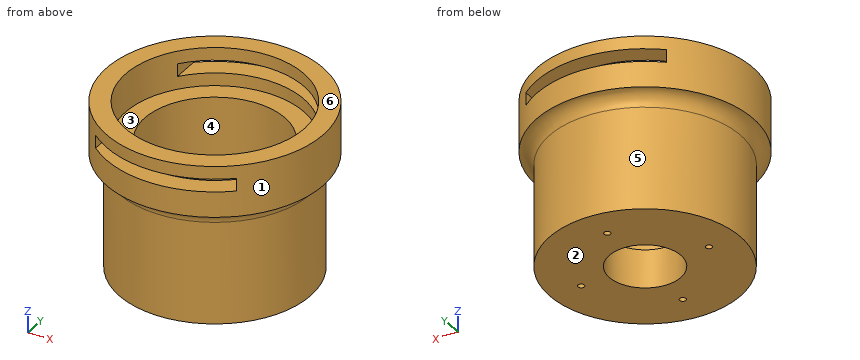
```python
from build123d import *

# Parameters (mm, degrees)
SKETCH1_R                = 15
BOSS_EXTRUDE5_DEPTH      = 26
SKETCH3_R                = 5.625
CUT_EXTRUDE2_DEPTH       = 34.555923471
CUT_EXTRUDE3_DEPTH       = 28
CUT_EXTRUDE3_DEPTH_BACK  = 20
SKETCH4_R                = 11
CUT_EXTRUDE6_START       = 6
SKETCH7_R                = 11
SKETCH7_R_2              = 9
CUT_EXTRUDE6_DEPTH       = 2
BOSS_EXTRUDE8_DEPTH      = 6
BOSS_EXTRUDE8_DEPTH_BACK = 2
BOSS_EXTRUDE8_START      = 20
SKETCH12_R               = 17
CUT_EXTRUDE10_START      = 18
SKETCH13_R               = 11
CUT_EXTRUDE10_DEPTH      = 18.411862419
FILLET2_R                = 2
CUT_EXTRUDE11_START      = 26
SKETCH14_R               = 14
CUT_EXTRUDE11_DEPTH      = 6
SKETCH15_R               = 0.5
CUT_EXTRUDE14_DEPTH      = 36.411862419
CUT_EXTRUDE15_DEPTH      = 36.411862419
CUT_EXTRUDE15_DEPTH_BACK = 36.411862419
SKETCH18_W               = 22
SKETCH18_H               = 2


with BuildPart() as part:
    # Sketch1 → Boss-Extrude5 (new body)
    with BuildSketch(Plane.XY):
        Circle(SKETCH1_R)
    extrude(amount=BOSS_EXTRUDE5_DEPTH)

    # Sketch3 → Cut-Extrude2 (cut, through all)
    with BuildSketch(Plane.XY.offset(26)):
        Circle(SKETCH3_R)
    extrude(amount=-CUT_EXTRUDE2_DEPTH, mode=Mode.SUBTRACT)

    # Sketch4 → Cut-Extrude3 (cut, two sides: drawn at the far end of the back side and taken through both)
    with BuildSketch(Plane.XY.offset(26).offset(-CUT_EXTRUDE3_DEPTH_BACK)):
        Circle(SKETCH4_R)
    extrude(amount=CUT_EXTRUDE3_DEPTH + CUT_EXTRUDE3_DEPTH_BACK, mode=Mode.SUBTRACT)

    # Sketch7 → Cut-Extrude6 (cut)
    with BuildSketch(Plane.XY.offset(CUT_EXTRUDE6_START)):
        Circle(SKETCH7_R)
        Circle(SKETCH7_R_2, mode=Mode.SUBTRACT)
    extrude(amount=-CUT_EXTRUDE6_DEPTH, mode=Mode.SUBTRACT)

    # Sketch12 → Boss-Extrude8 (add, two sides: drawn at the far end of the back side and taken through both)
    with BuildSketch(Plane.XY.offset(BOSS_EXTRUDE8_START - BOSS_EXTRUDE8_DEPTH_BACK)):
        Circle(SKETCH12_R)
    extrude(amount=BOSS_EXTRUDE8_DEPTH + BOSS_EXTRUDE8_DEPTH_BACK)

    # Sketch13 → Cut-Extrude10 (cut, through all)
    with BuildSketch(Plane.XY.offset(CUT_EXTRUDE10_START)):
        Circle(SKETCH13_R)
    extrude(amount=CUT_EXTRUDE10_DEPTH, mode=Mode.SUBTRACT)

    # Fillet2
    fillet2_edges = [part.edges().sort_by_distance(p)[0] for p in [
        (-15, 0, 18),
    ]]
    fillet(fillet2_edges, radius=FILLET2_R - 0.0001)  # a hair under: the kernel refuses the full size

    # Sketch14 → Cut-Extrude11 (cut)
    with BuildSketch(Plane.XY.offset(CUT_EXTRUDE11_START)):
        Circle(SKETCH14_R)
    extrude(amount=-CUT_EXTRUDE11_DEPTH, mode=Mode.SUBTRACT)

    # Sketch15 → Cut-Extrude14 (cut, through all)
    with BuildSketch(Plane.XY):
        with Locations((0, 10)):
            Circle(SKETCH15_R)
        with Locations((0, -10)):
            Circle(SKETCH15_R)
        with Locations((10, 0)):
            Circle(SKETCH15_R)
        with Locations((-10, 0)):
            Circle(SKETCH15_R)
    extrude(amount=CUT_EXTRUDE14_DEPTH, mode=Mode.SUBTRACT)

    # Sketch18 → Cut-Extrude15 (cut, two sides: drawn at the far end of the back side and taken through both)
    with BuildSketch(Plane(origin=(0, 0, 0), x_dir=(1, 0, 0), z_dir=(0, 1, 0)).offset(-CUT_EXTRUDE15_DEPTH_BACK)):
        with Locations((0, -23)):
            Rectangle(SKETCH18_W, SKETCH18_H)
    extrude(amount=CUT_EXTRUDE15_DEPTH + CUT_EXTRUDE15_DEPTH_BACK, mode=Mode.SUBTRACT)


solid = part.part
```
Input: part model. Units: mm. Frame: model coordinates. Face numbers are marked on the shaded views. A direction names the side the tool comes from. Give positions to 0.01 mm unless a question says otherwise; leave off trailing zeros. Order: outer loops, then holes, each group sorted by start corner. A loop starts at its lowest first (then second) coordinate and runs counter-clockwise, first axis right, second up.
1. Section B-B on z = 2.5. Return the cut outline in (x, y) (3 decimals), and give its area (3 significant figures).
Derived:
outline: circle Ø30 at (0, 0); hole circle Ø1 at (-10, 0); hole circle Ø11.25 at (0, 0); hole circle Ø1 at (0, -10); hole circle Ø1 at (0, 10); hole circle Ø1 at (10, 0)
area: 604 mm2
2. Mould query, pull axis Y, two halves, no side actions, for the marked faces 1, 2 and 3. Classes: released by +Y, released by -Y, zero draft, split by the parting line, or undercut.
Derived:
face 1: split by the parting line
face 2: zero draft
face 3: undercut
3. Section D-D on z = 8.5. Return the cut outline in (x, y), and give its area (3 significant figures).
Derived:
outline: circle Ø30 at (0, 0); hole circle Ø22 at (0, 0)
area: 327 mm2
4. Section A-A on y = 0. Give the number of separate pieces and of enclosed holes in the cut face, and give its area (3 significant figures).
Derived:
separate pieces: 4
enclosed holes: 0
area: 254 mm2
5. Material intervals for L1, parallel to Y at x = 0, z = 4.25 (3 decimals); L2, parallel to Y at x = 0, z = 2.25 (3 decimals); L3, parallel to X at y = 0, z = 10.5, sorted ascending.
Derived:
L1: y = -15 to -11, -9 to -5.625, 5.625 to 9, 11 to 15
L2: y = -15 to -10.5, -9.5 to -5.625, 5.625 to 9.5, 10.5 to 15
L3: x = -15 to -11, 11 to 15
6. Reachability of the marked faces 4, 5 and 6 from +Z, -Z, +X, -X, +Y, -Y: full face, straight path, thin tool, end or side. Return the list, or none.
Derived:
face 4: +Z
face 5: -Z
face 6: +Z, +X, -X, +Y, -Y
7. Pin query (flat end, axial travel): pin 1 (14.5 mm diameter, centred on x = 1.5, y = 0, fed in from +Z); pin 2 (4 mm diameter, centred on x = -3.5, y = 11, fed in from -Z); pin 3 (2 mm diameter, centred on x = -3, z = 8, fed in from +Y); pin 4 (12 mm diameter, centred on x = 13.5, z = 5.5, fed in from +Y). Return the tip coordinate at first contact, or that it passes through.
Derived:
pin 1: stops at z = 6
pin 2: stops at z = 0
pin 3: stops at y = 14.87
pin 4: stops at y = 12.99
